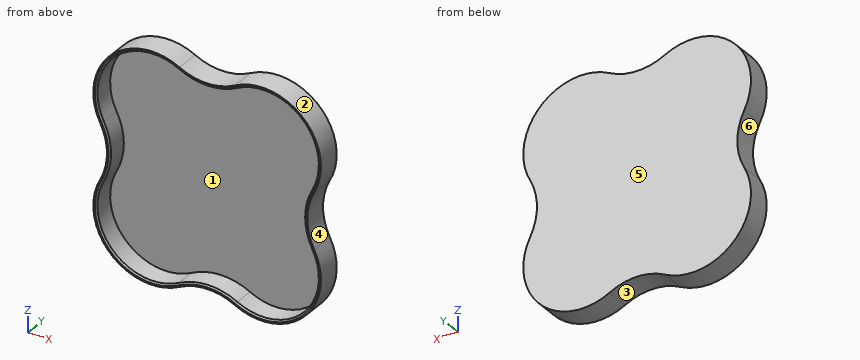
```python
from build123d import *

# Parameters (mm, degrees)
F1_DEPTH = 1
F3_DEPTH = 6.858
F4_SIZE  = 0.508


with BuildPart() as f1:
    # F0 (on Front) → F1 (new body)
    with BuildSketch(Plane.XZ):
        with BuildLine():
            ThreePointArc((-8.910079, 34.455263), (-31.114318, 31.114318), (-34.455263, 8.910079))
            ThreePointArc((-34.455263, 8.910079), (-32.243107, 0), (-34.455263, -8.910079))
            ThreePointArc((-34.455263, -8.910079), (-31.114318, -31.114318), (-8.910079, -34.455263))
            ThreePointArc((-8.910079, -34.455263), (0, -32.243107), (8.910079, -34.455263))
            ThreePointArc((8.910079, -34.455263), (31.114318, -31.114318), (34.455263, -8.910079))
            ThreePointArc((34.455263, -8.910079), (32.243107, 0), (34.455263, 8.910079))
            ThreePointArc((34.455263, 8.910079), (31.114318, 31.114318), (8.910079, 34.455263))
            ThreePointArc((8.910079, 34.455263), (0, 32.243107), (-8.910079, 34.455263))
        make_face()
    extrude(amount=F1_DEPTH)

    # F2 (on face) → F3 (join)
    with BuildSketch(Plane.XZ.offset(1)):
        with BuildLine():
            ThreePointArc((-8.910079, 34.455263), (-31.114318, 31.114318), (-34.455263, 8.910079))
            ThreePointArc((-34.455263, 8.910079), (-32.243107, 0), (-34.455263, -8.910079))
            ThreePointArc((-34.455263, -8.910079), (-31.114318, -31.114318), (-8.910079, -34.455263))
            ThreePointArc((-8.910079, -34.455263), (0, -32.243107), (8.910079, -34.455263))
            ThreePointArc((8.910079, -34.455263), (31.114318, -31.114318), (34.455263, -8.910079))
            ThreePointArc((34.455263, -8.910079), (32.243107, 0), (34.455263, 8.910079))
            ThreePointArc((34.455263, 8.910079), (31.114318, 31.114318), (8.910079, 34.455263))
            ThreePointArc((8.910079, 34.455263), (0, 32.243107), (-8.910079, 34.455263))
        make_face()
        with BuildLine():
            ThreePointArc((-33.571386, -9.3778), (-31.243107, 0), (-33.571386, 9.3778))
            ThreePointArc((-33.571386, 9.3778), (-30.407211, 30.407211), (-9.3778, 33.571386))
            ThreePointArc((-9.3778, 33.571386), (0, 31.243107), (9.3778, 33.571386))
            ThreePointArc((9.3778, 33.571386), (30.407211, 30.407211), (33.571386, 9.3778))
            ThreePointArc((33.571386, 9.3778), (31.243107, 0), (33.571386, -9.3778))
            ThreePointArc((33.571386, -9.3778), (30.407211, -30.407211), (9.3778, -33.571386))
            ThreePointArc((9.3778, -33.571386), (0, -31.243107), (-9.3778, -33.571386))
            ThreePointArc((-9.3778, -33.571386), (-30.407211, -30.407211), (-33.571386, -9.3778))
        make_face(mode=Mode.SUBTRACT)
    extrude(amount=F3_DEPTH)

    # F4
    f4_edges = [f1.edges().sort_by_distance(p)[0] for p in [
        (-30.407211, -7.858, 30.407211),
    ]]
    chamfer(f4_edges, length=F4_SIZE)


solid = f1.part
```
Build history of the part. All positions in model axes, mm. Face numbers are marked on the shaded views. A direction names the side the tool comes from. Coordinates: 2 decimals unless noted, no trailing zeros. Write each loop counter-clockwise with the first axis right and the second up, starting at its lowest first coordinate (ties: lowest second). Pieces come first, ordered by that corner, then holes.
1. Drill centre lines: probe 1 along Z at (x, y) = (-34, -5.5); probe 2 along Y at (x, z) = (9, 11). Where is each one in solid material? Low to high.
Answer block:
probe 1: z = -27.4 to -25.26, -10.24 to -7.99, 7.99 to 10.24, 25.26 to 27.4
probe 2: y = -1 to 0
2. Pull direction X, two halves, no side cores. Call the marked faces 3, 4, 5 and 6: released by +X, released by -X, zero draft, split by the parting line, or undercut.
Answer block:
face 3: undercut
face 4: released by +X
face 5: zero draft
face 6: released by -X
3. 3-axis set-ups, long thin cutter, end or side, ignore diameter. For the marked faces 1 and 2: which of +Z, -Z, +X, -X, +Y, -Y reach the whole face in a straight line?
Answer block:
face 1: -Y
face 2: +Y, -Y
4. Drop flat-ended pins along their axis: pin 1 (3 mm diameter, centred on x = -13, y = -3.5, fed in from -Z); pin 2 (5 mm diameter, centred on x = -22.5, z = 2.5, fed in from -Y); pin 3 (2 mm diameter, centred on y = -6.5, z = 25.5, fed in from +X). Give the stop position or say it passes through.
Answer block:
pin 1: stops at z = -36.37
pin 2: stops at y = -1
pin 3: stops at x = 35.4
5. Band-saw the part on A-A, the plane y = -5.75. Give the cut face in (x, z).
Answer block:
outline: (-34.46, -8.91) arc R18.9 ccw to (-8.91, -34.46) arc R19.05 cw to (8.91, -34.46) arc R18.9 ccw to (34.46, -8.91) arc R19.05 cw to (34.46, 8.91) arc R18.9 ccw to (8.91, 34.46) arc R19.05 cw to (-8.91, 34.46) arc R18.9 ccw to (-34.46, 8.91) arc R19.05 cw to start; hole (-33.57, -9.38) arc R17.9 ccw to (-9.38, -33.57) arc R20.05 cw to (9.38, -33.57) arc R17.9 ccw to (33.57, -9.38) arc R20.05 cw to (33.57, 9.38) arc R17.9 ccw to (9.38, 33.57) arc R20.05 cw to (-9.38, 33.57) arc R17.9 ccw to (-33.57, 9.38) arc R20.05 cw to start
